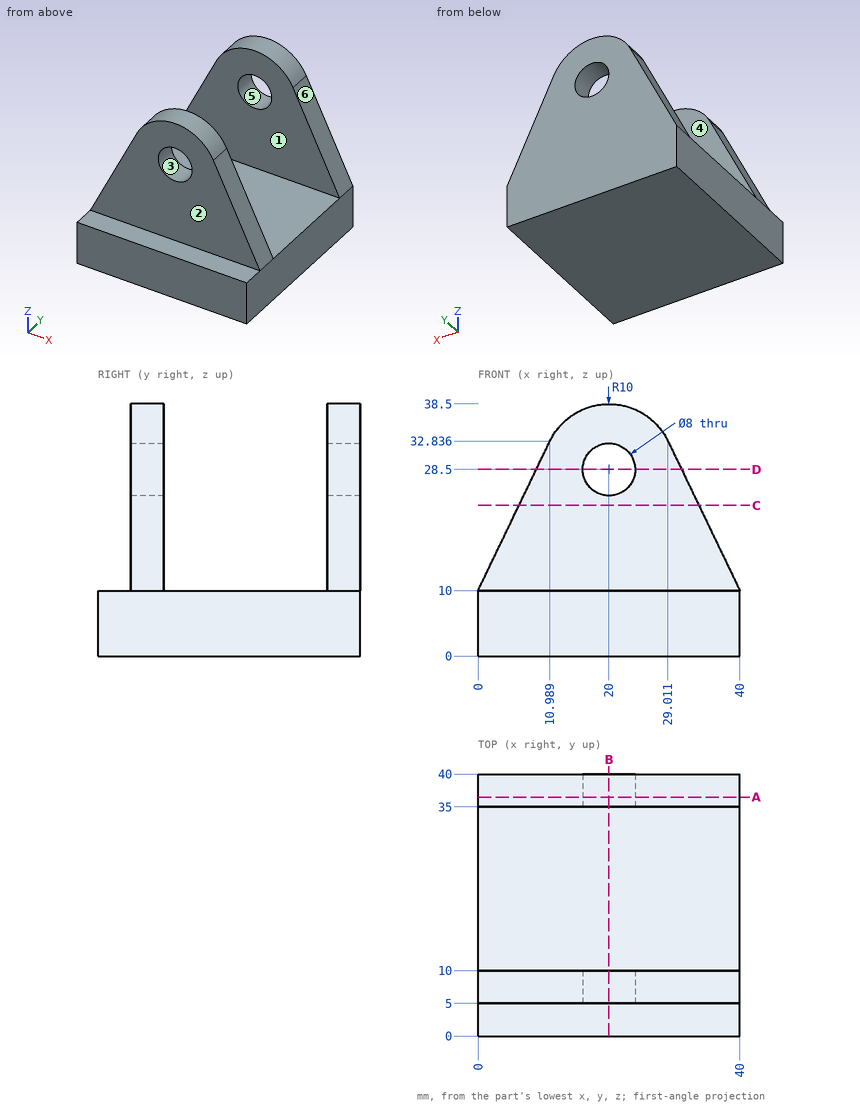
Source: three-view drawing plus pictorial views. Frame: mm from the lowest corner of the part. A direction names the side the tool comes from. Round coordinates to 2 decimals unless told otherwise and drop trailing zeros. Write each loop counter-clockwise with the first axis right and the second up, starting at its lowest first coordinate (ties: lowest second). Pieces come first, ordered by that corner, then holes. Notation, with made-up numbers: (-10, 13.25) -> (49, 13.25) arc R21 cw to (49, 37.25) -> close; hole circle Ø10 at (73, 27). An arc over 180 degrees is marked (long way). Return JSON: item names as keys, results as strings.
Q1. First-contact query: pin 1 Ø8.5 at (x, z) = (18, 21.5) entering from -Y; pin 2 Ø5.5 at (x, y) = (20, 1.5) entering from +Z; pin 3 Ø5 at (x, z) = (20, 28.5) entering from +Y; pin 4 Ø6 at (x, y) = (24.5, 35) entering from +Z. Flat tips, straight axial feed; report the tip coordinate or a pass-through.
From the geometry:
{"pin 1": "y = 5", "pin 2": "z = 10", "pin 3": "through", "pin 4": "z = 38.39"}
Q2. Section B-B on x = 20. Return the cut outline in (y, z).
From the geometry:
{"outline": "(0, 0) -> (40, 0) -> (40, 24.5) -> (35, 24.5) -> (35, 10) -> (10, 10) -> (10, 24.5) -> (5, 24.5) -> (5, 10) -> (0, 10) -> close; (5, 32.5) -> (10, 32.5) -> (10, 38.5) -> (5, 38.5) -> close; (35, 32.5) -> (40, 32.5) -> (40, 38.5) -> (35, 38.5) -> close"}
Q3. Mould query, pull axis X, two halves, no side actions, for the marked faces 4, 5 and 6. Classes: +X half, -X half, draft (parallel to the pull), parting line (faces both ways), or undercut.
From the geometry:
{"face 4": "draft", "face 5": "undercut", "face 6": "+X half"}
Q4. Section C-C on z = 23. Return the cut outline in (x, y).
From the geometry:
{"outline": "(6.26, 5) -> (33.74, 5) -> (33.74, 10) -> (6.26, 10) -> close; (6.26, 35) -> (33.74, 35) -> (33.74, 40) -> (6.26, 40) -> close"}
Q5. Section D-D on z = 28.5. Return the cut outline in (x, y).
From the geometry:
{"outline": "(8.9, 5) -> (16, 5) -> (16, 10) -> (8.9, 10) -> close; (8.9, 35) -> (16, 35) -> (16, 40) -> (8.9, 40) -> close; (24, 5) -> (31.1, 5) -> (31.1, 10) -> (24, 10) -> close; (24, 35) -> (31.1, 35) -> (31.1, 40) -> (24, 40) -> close"}
Q6. Set-up query: the marked faces 1, 2 and 3. Return all of +Z, -Z, +X, -X, +Y, -Y with unobstructed straight access to the full face (end or side cutting, diameter ignored); none if empty.
From the geometry:
{"face 1": "+Z, +X, -X", "face 2": "+Z, +X, -X, -Y", "face 3": "+Y, -Y"}
Q7. Section A-A on y = 36.5. Return the cut outline in (x, z).
From the geometry:
{"outline": "(0, 0) -> (40, 0) -> (40, 10) -> (29.01, 32.84) arc R10 ccw to (10.99, 32.84) -> (0, 10) -> close; hole circle Ø8 at (20, 28.5)"}
Q8. Ray query, line 1 (Y direction, x = 34, z = 16); line 2 (Z direction, x = 13.5, y = 24.5); line 3 (X direction, y = 7.25, z = 28.5). Return the intervals inside material, ascending.
From the geometry:
{"line 1": "5 to 10, 35 to 40", "line 2": "0 to 10", "line 3": "8.9 to 16, 24 to 31.1"}
